Design review of the part built by this model. Coordinates are the model's own, in mm. Give positions to 0.01 mm unless a question says otherwise; leave off trailing zeros. Order: outer loops, then holes, each group sorted by start corner. A loop starts at its lowest first (then second) coordinate and runs counter-clockwise, first axis right, second up. Notation, with made-up numbers: (-34.75, 77) -> (-10.75, 77) arc R17 ccw to (-10.75, 103) -> close; hole circle Ø9 at (40.5, 47.25). An arc over 180 degrees is marked (long way). Return JSON: item names as keys, results as strings.
```python
from build123d import *

# Parameters (mm, degrees)
EXTRUDE_2_DEPTH               = 100
HOLE_WIZARD_M60_2_D           = 54.5
HOLE_WIZARD_M60_2_CSINK_D     = 60.05
HOLE_WIZARD_M60_2_CSINK_ANGLE = 90


with BuildPart() as part:
    # 草图1 → 凸台-拉伸2 (new body)
    with BuildSketch(Plane(origin=(0, 0, 0), x_dir=(1, 0, 0), z_dir=(0, 1, 0))):
        with BuildLine():
            ThreePointArc((33, 11.66190379), (0, 35), (-33, 11.66190379))
            Line((-33, 11.66190379), (-33, -11.66190379))
            ThreePointArc((-33, -11.66190379), (0, -35), (33, -11.66190379))
            Line((33, -11.66190379), (33, 11.66190379))
        make_face()
    extrude(amount=EXTRUDE_2_DEPTH)

    # M60 螺纹孔2 (through all)
    with Locations(Plane.ZX.offset(100)):
        with Locations((0, 0)):
            CounterSinkHole(HOLE_WIZARD_M60_2_D / 2, HOLE_WIZARD_M60_2_CSINK_D / 2, counter_sink_angle=HOLE_WIZARD_M60_2_CSINK_ANGLE)


solid = part.part
```
Item 1: Add section A-A (x = 0). Give the boundary of the cut face in (y, z) (3 decimals).
Result set:
{"outline": "(0, -35) -> (100, -35) -> (100, -30.025) -> (97.225, -27.25) -> (0, -27.25) -> close; (0, 27.25) -> (97.225, 27.25) -> (100, 30.025) -> (100, 35) -> (0, 35) -> close"}
Item 2: Mouldability with a two-part tool opening along Z and no side actions: class faces 1 (the face through (8.23, 97.36, -26.12)), 2 (the face through (0.603, 49.3, -34.995)), 3 (the face through (33, 49, 0)) as released by +Z, released by -Z, zero draft, split by the parting line, or undercut.
Result set:
{"face 1": "undercut", "face 2": "released by -Z", "face 3": "zero draft"}
Item 3: For pin 1 (3 mm diameter, centred on x = -5, y = 74, fed in from -Z); pin 2 (2 mm diameter, centred on x = -21.5, y = 54.5, fed in from +Z); pin 3 (2 mm diameter, centred on x = 21, y = 88, fed in from +Z), all flat-tipped, find the tip position at first contact; note any pin that passes through.
Result set:
{"pin 1": "stops at z = -34.82", "pin 2": "stops at z = 28.37", "pin 3": "stops at z = 28.72"}
Item 4: Wall thickness on L1, parallel to Z at x = 0, y = 44.5; L2, parallel to X at y = 70, z = 0; L3, parallel to Z at x = 9, y = 93.5: over which ranges is each line inside the solid? List them lowest first. Write a range as [from, to].
Result set:
{"L1": "z = [-35, -27.25], [27.25, 35]", "L2": "x = [-33, -27.25], [27.25, 33]", "L3": "z = [-33.82, -25.72], [25.72, 33.82]"}
Item 5: Add section B-B (y = 47.5). Give the boundary of the cut face in (x, z).
Result set:
{"outline": "(-33, -11.66) arc R35 ccw to (33, -11.66) -> (33, 11.66) arc R35 ccw to (-33, 11.66) -> close; hole circle Ø54.5 at (0, 0)"}
Item 6: Add section C-C (z = 0). Give the boundary of the cut face in (x, y) (3 decimals), plus the area to 3 significant figures.
Result set:
{"outline": "(-33, 0) -> (-27.25, 0) -> (-27.25, 97.225) -> (-30.025, 100) -> (-33, 100) -> close; (27.25, 0) -> (33, 0) -> (33, 100) -> (30.025, 100) -> (27.25, 97.225) -> close", "area": "1,140 mm^2"}
